CAD build for the part. Positions are in the model's coordinates, mm. A direction names the side the tool comes from. Give positions to 0.01 mm unless a question says otherwise; leave off trailing zeros. Write each loop counter-clockwise with the first axis right and the second up, starting at its lowest first coordinate (ties: lowest second). Pieces come first, ordered by that corner, then holes. Notation, with made-up numbers: (-31, 14) -> (1, 14) arc R16 ccw to (1, 21) -> close; hole circle Ø1 at (4, 28). An arc over 180 degrees is marked (long way). Use one line per item in the form item = value. Start each with the question number.
Autodesk Inventor part; units mm, degrees
ref_plane "YZ Plane" through (0, 0, 0) normal (1, 0, 0) x (0, 1, 0)
ref_plane "XZ Plane" through (0, 0, 0) normal (0, 1, 0) x (-1, 0, 0)
ref_plane "XY Plane" through (0, 0, 0) normal (0, 0, 1) x (1, 0, 0)
sketch "Skizze1" plane through (0, 0, 0) normal (1, 0, 0) x (0, 1, 0)
  arc A0 (-6.9821, 8.5) -> (6.9821, 8.5) centre (0, 0) ccw construction
  line L0 (14, 8.5) -> (-14, 8.5)
  line L1 (-14, 8.5) -> (-14, 0.8162)
  line L2 (0, 12.4) -> (0, -14.9)
  circle A1 centre (0, 0) radius 5
  line L3 (14, 0.8162) -> (14, 8.5)
  line L4 (-14, 0.8162) -> (-5.7262, -11)
  line L5 (-5.7262, -11) -> (5.7262, -11)
  line L6 (5.7262, -11) -> (14, 0.8162)
  circle A2 centre (10.009, -1.351) radius 1.1
  circle A3 centre (-10.009, -1.351) radius 1.1
  dimension "d0" = 22
  dimension "d2" = 10
  dimension "d19" = 8.5
  dimension "d39" = 14
  dimension "d50" = 2.2
  dimension "d57" = 10.009
  dimension "d58" = 1.351
  dimension "d59" = 35
extrude "Extrusion1" add sketch "Skizze1" along normal mid plane 6 contours L3 L6 L5 L2 A1 L0 | L2 A1 L5 L4 L1 L0
sketch "Skizze2" plane through (3, 0, 0) normal (1, 0, 0) x (0, 0, -1)
  circle A0 centre (0, 0) radius 8.5 construction
  line L0 (0, 0) -> (8.5, 0) construction
  line L1 (-12.4, 0) -> (14.9, 0)
  dimension "d6" = 17
hole "Bohrung1" at (3, 0, -8.5) direction (-1, 0, 0) diameter 2.1 end through all counterbore diameter 4.2 counterbore depth 2.8
pattern_circular "Runde Anordnung1" count 3 over 360 about axis through (0, 0, 0) along (1, 0, 0) of "Bohrung1"
sketch "Skizze3" plane through (-3, -14, 8.5) normal (0, 0, 1) x (1, 0, 0)
  line L0 (0, 0) -> (6, 0)
  line L1 (6, 28) -> (6, 0)
  line L2 (0, 0) -> (0, 28)
  line L3 (0, 0) -> (6, 0) construction
  line L4 (3, 0) -> (3, 24.0467) construction
  line L5 (6, 28) -> (0, 28)
  line L6 (-1.2, 14) -> (7.2, 14)
  point P0 (3, 14)
  point P1 (3, 3)
  point P2 (3, 25)
  dimension "d44" = 11
hole "Bohrung2" at (0, -11, 8.5) at (0, 11, 8.5) direction (0, 0, -1) diameter 2.459 depth 7 tip angle 118
sketch "Skizze5" plane through (3, 0, 0) normal (1, 0, 0) x (0, 0, -1)
  circle A0 centre (0, 0) radius 6.5
  dimension "d41" = 13
extrude "Extrusion2" [suppressed]
chamfer "Fase1" [suppressed]
fillet "Rundung2" radius 2 4 edges at (0, -5.7262, -11) (0, 5.7262, -11) (0, -14, 0.8162) (0, 14, 0.8162)
fillet "Rundung1" [suppressed]
properties part number "Motorhalter" material "Aluminium 6061"
1) Wall check: line 1 along Z through (x, y) = (1.55, 0); line 2 along X through (y, z) = (-11, 7.75); line 3 along Y through (x, z) = (-1.05, 4). Give the ranges that are in metal, low to high. Write a range as from..to.
2) Cut at D-D (z = -4.5). Give the cut face in (x, y), and give its area (3 significant figures).
3) Two-plate mould, pull along Z, no slides. Class faces 3 (the face through (1.58, -0.09, -6.4)), 4 (the face through (0, 14, 5)), 5 (the face through (0.2, 0.9, -9.4)), 6 (the face through (0.04, -13.91, 0.85)): released by +Z, released by -Z, zero draft, split by the parting line, or undercut.
4) Pin check, flat tips, straight feed: pin 1 (2.5 mm diameter, centred on y = 7.36, z = 4.25, fed in from -X); pin 2 (3.5 mm diameter, centred on y = 0, z = -8.5, fed in from +X); pin 3 (1.5 mm diameter, centred on x = 2, z = -2.5, fed in from -Y); pin 4 (2 mm diameter, centred on x = -2.5, y = 6, fed in from -Z). Stop position of each tip, or through.
5) Cut at A-A (z = 4.25). Give the cut face in (x, y).
6) Cut at B-B (y = -3). Give the cut face in (x, z), and give its area (3 significant figures).
7) Cut at C-C (y = 0). Give the cut face in (x, z).
8) 3-axis set-ups, long thin cutter, end or side, ignore diameter. For faces 1 (the face through (-0.04, 5.62, -10.77)), 2 (the face through (1.58, 8.639, 5.916)): which of +Z, -Z, +X, -X, +Y, -Y reach the whole face in a straight line?
Final values:
q1.line_1 = -11..-10.6, -6.4..-5, 5..8.5
q1.line_2 = -3..-1.23, 1.23..3
q1.line_3 = -14..-11.64, -10.36..-8.38, -6.34..-3, 3..6.34, 8.38..10.36, 11.64..14
q2.outline = (-3, -10.28) -> (3, -10.28) -> (3, -2.18) -> (-3, -2.18) -> close; (-3, 2.18) -> (3, 2.18) -> (3, 10.28) -> (-3, 10.28) -> close
q2.area = 97.2 mm^2
q3.face_3 = undercut
q3.face_4 = zero draft
q3.face_5 = undercut
q3.face_6 = released by -Z
q4.pin_1 = -3
q4.pin_2 = 0.2
q4.pin_3 = -12.2
q4.pin_4 = -10.98
q5.outline = (-3, -14) -> (3, -14) -> (3, -9.46) -> (0.2, -9.46) -> (0.2, -8.41) -> (-3, -8.41) -> close; (-3, -6.31) -> (0.2, -6.31) -> (0.2, -5.26) -> (3, -5.26) -> (3, -2.63) -> (-3, -2.63) -> close; (-3, 2.63) -> (3, 2.63) -> (3, 5.26) -> (0.2, 5.26) -> (0.2, 6.31) -> (-3, 6.31) -> close; (-3, 8.41) -> (0.2, 8.41) -> (0.2, 9.46) -> (3, 9.46) -> (3, 14) -> (-3, 14) -> close; hole circle Ø2.46 at (0, -11); hole circle Ø2.46 at (0, 11)
q6.outline = (-3, -11) -> (3, -11) -> (3, -4) -> (-3, -4) -> close; (-3, 4) -> (3, 4) -> (3, 8.5) -> (-3, 8.5) -> close
q6.area = 69.0 mm^2
q7.outline = (-3, -11) -> (3, -11) -> (3, -10.6) -> (0.2, -10.6) -> (0.2, -9.55) -> (-3, -9.55) -> close; (-3, -7.45) -> (0.2, -7.45) -> (0.2, -6.4) -> (3, -6.4) -> (3, -5) -> (-3, -5) -> close; (-3, 5) -> (3, 5) -> (3, 8.5) -> (-3, 8.5) -> close
q8.face_1 = -Z, +X, -X, +Y
q8.face_2 = +X
